Geometry check sheet. Reference: drawing and pictorial views, mm from the part's lowest x, y, z. A direction names the side the tool comes from. Give positions to 0.01 mm unless a question says otherwise; leave off trailing zeros. Loops run counter-clockwise (first coordinate to the right, second up) from the corner with the lowest first, then second, coordinate; pieces in that order, holes last. Notation, with made-up numbers: (-32.5, 75.5) - (-15.5, 75.5) arc R13 cw to (-15.5, 85.5) - close; hole circle Ø11 at (48.5, 28.5). An arc over 180 degrees is marked (long way). One line per question, with ' | ' between items. Start each with the question number.
1. Section check B-B, the plane y = 24. Enter the section's corners in (x, z).
2. Section check A-A, the plane x = 11. Enter the section's corners in (y, z).
3. Depth check by flat-ended pin: pin 1 Ø24 at (x, y) = (26, 29) entering from +Z; pin 2 Ø4.5 at (x, y) = (3, 24) entering from +Z; pin 3 Ø2 at (y, z) = (21, 11.5) entering from -X; pin 4 Ø7 at (y, z) = (42.5, 10) entering from +X. Enter the tip coordinate at first touch or a pass-through.
4. Thickness scan on line 1 along Y through (x, z) = (16.5, 6.5); line 2 along Z through (x, y) = (36.2, 7.5); line 3 along X through (y, z) = (26, 9.75). Record the ranges inside material, lowest first. Write a range as from..to.
5. Tool access check on the marked faces 1, 2 and 3. Record the directions out of +Z, -Z, +X, -X, +Y, -Y that give a thin tool (end or side, any length) a straight path to the whole face; none if there is none.
6. Section check C-C, the plane z = 11.25. State how many separate pieces and enclosed holes the cut face has, then the cut area to 3 significant figures.
7. Section check D-D, the plane z = 16.5. Enter the section's corners in (x, y).
8. Mould release check, pull along Z, two halves, no side actions. Record for the marked faces 4, 5 and 6: +Z half, -Z half, draft (parallel to the pull), parting line (faces both ways), or undercut.
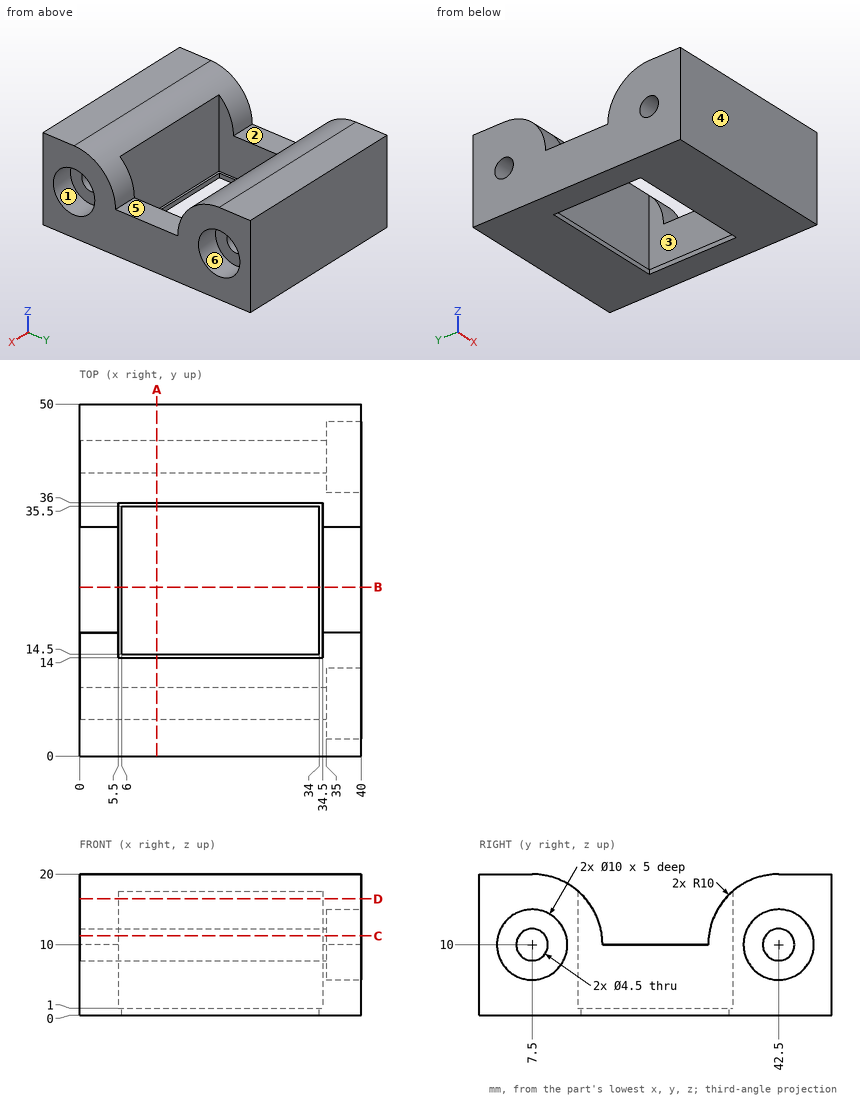
Results list:
1) outline: (0, 0) - (6, 0) - (6, 1) - (5.5, 1) - (5.5, 10) - (0, 10) - close; (34, 0) - (40, 0) - (40, 10) - (34.5, 10) - (34.5, 1) - (34, 1) - close
2) outline: (0, 0) - (14.5, 0) - (14.5, 1) - (14, 1) - (14, 17.6) arc R10 ccw to (7.5, 20) - (0, 20) - close; (35.5, 0) - (50, 0) - (50, 20) - (42.5, 20) arc R10 ccw to (36, 17.6) - (36, 1) - (35.5, 1) - close; hole circle Ø4.5 at (7.5, 10); hole circle Ø4.5 at (42.5, 10)
3) pin 1: z = 19.89 | pin 2: z = 10 | pin 3: through | pin 4: x = 35
4) line 1: 0..14, 36..50 | line 2: 0..5, 15..20 | line 3: 0..5.5, 34.5..40
5) face 1: +X | face 2: +Z, +X, -X | face 3: +Z
6) separate pieces: 4 | enclosed holes: 0 | area: 837 mm²
7) outline: (0, 0) - (40, 0) - (40, 15.1) - (34.5, 15.1) - (34.5, 14) - (5.5, 14) - (5.5, 15.1) - (0, 15.1) - close; (0, 34.9) - (5.5, 34.9) - (5.5, 36) - (34.5, 36) - (34.5, 34.9) - (40, 34.9) - (40, 50) - (0, 50) - close
8) face 4: draft | face 5: +Z half | face 6: undercut
